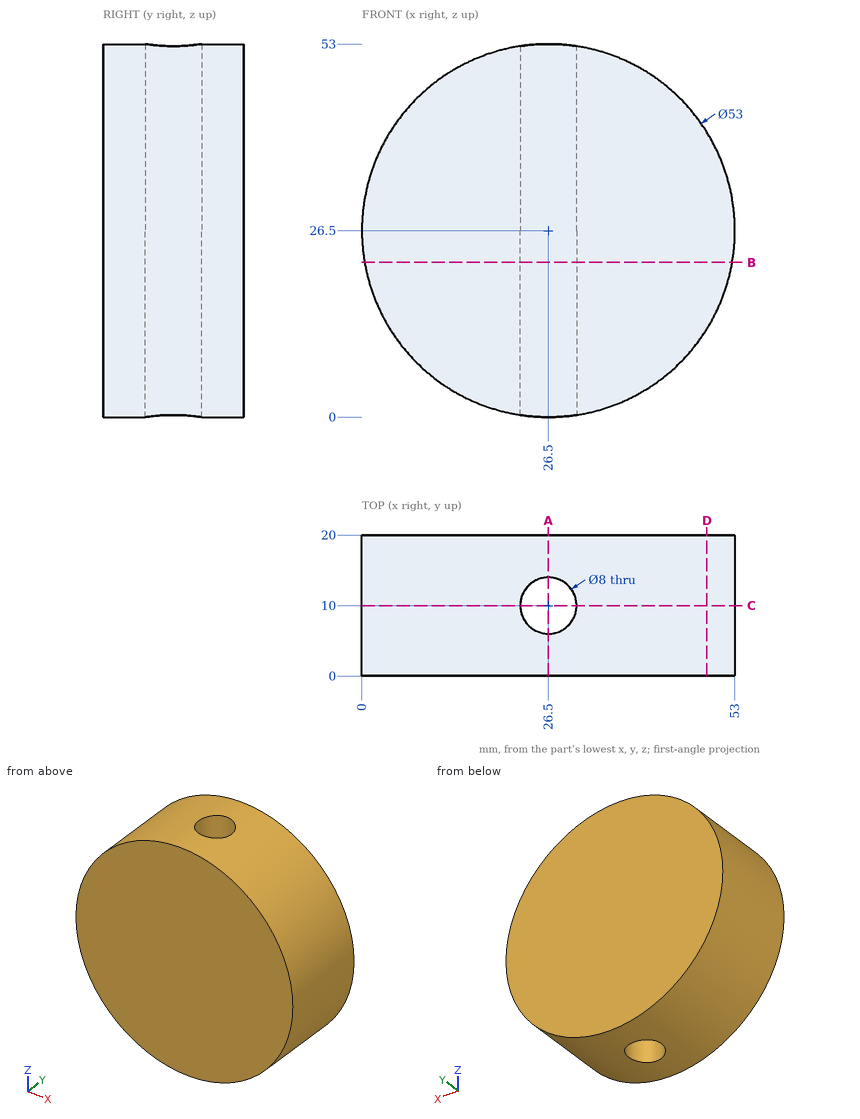
Job drawing, mm, ordinate dimensions from the low corner. One solid piece. Coordinates: 2 decimals unless noted, no trailing zeros. Order: outer loops, then holes, each group sorted by start corner. A loop starts at its lowest first (then second) coordinate and runs counter-clockwise, first axis right, second up. Notation, with made-up numbers: (89, 21.5) - (123, 21.5) arc R17 ccw to (123, 34.5) - close; hole circle Ø1 at (25.5, 60.25). An arc over 180 degrees is marked (long way). Write each question's results on one line, items separated by ' | '. Start each with the question number.
Item 1: Flat gauge pins, fed straight in: pin 1 (1.5 mm diameter, centred on y = 13, z = 20.5, fed in from +X); pin 2 (4 mm diameter, centred on x = 45, y = 13, fed in from -Z); pin 3 (3 mm diameter, centred on y = 2.5, z = 29.5, fed in from +X). Where does each tip first touch, or does it go through?
Item 2: Band-saw the part on C-C on y = 10. Write the cut outline in (x, z).
Item 3: Band-saw the part on A-A on x = 26.5. Write the cut outline in (y, z).
Item 4: Band-saw the part on D-D on x = 49. Write the cut outline in (y, z), and give its area (3 significant figures).
Item 5: Band-saw the part on B-B on z = 22. Write the cut outline in (x, y), and give its area (3 significant figures).
Item 6: Wall check: probe 1 along Y at (x, z) = (26.5, 10.75); probe 2 along X at (y, z) = (11, 17.5); probe 3 along X at (y, z) = (8.25, 37.5). Give the ranges that are in metal, low to high. Write a range as [from, to].
Numbers:
1) pin 1: x = 52.47 | pin 2: z = 5.76 | pin 3: x = 52.96
2) outline: (22.5, 0.3) - (22.5, 52.7) arc R26.5 ccw to start; (30.5, 0.3) arc R26.5 ccw to (30.5, 52.7) - close
3) outline: (0, 0) - (6, 0) - (6, 53) - (0, 53) - close; (14, 0) - (20, 0) - (20, 53) - (14, 53) - close
4) outline: (0, 12.5) - (20, 12.5) - (20, 40.5) - (0, 40.5) - close | area: 560 mm^2
5) outline: (0.38, 0) - (52.62, 0) - (52.62, 20) - (0.38, 20) - close; hole circle Ø8 at (26.5, 10) | area: 994 mm^2
6) probe 1: [0, 6], [14, 20] | probe 2: [1.58, 22.63], [30.37, 51.42] | probe 3: [2.39, 22.9], [30.1, 50.61]
